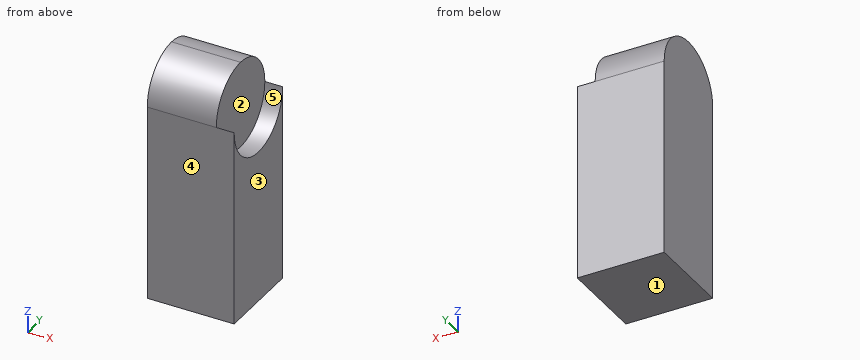
from build123d import *

# Parameters (mm, degrees)
SKETCH2_W           = 17
SKETCH2_H           = 17
BOSS_EXTRUDE1_DEPTH = 47
CUT_EXTRUDE1_DEPTH  = 47
SKETCH6_R           = 8.5
CUT_EXTRUDE3_DEPTH  = 3.5


with BuildPart() as part:
    # Sketch2 → Boss-Extrude1 (new body)
    with BuildSketch(Plane.XY):
        Rectangle(SKETCH2_W, SKETCH2_H)
    extrude(amount=BOSS_EXTRUDE1_DEPTH)

    # Sketch3 → Cut-Extrude1 (cut)
    with BuildSketch(Plane(origin=(8.5, 0, 0), x_dir=(0, 0, -1), z_dir=(1, 0, 0))):
        with BuildLine():
            Line((-38.5, 8.5), (-47, 8.5))
            Line((-47, 8.5), (-47, 0))
            ThreePointArc((-47, 0), (-44.51040764, 6.01040764), (-38.5, 8.5))
        make_face()
        with BuildLine():
            ThreePointArc((-38.5, -8.5), (-44.51040764, -6.01040764), (-47, 0))
            Line((-47, 0), (-47, -8.5))
            Line((-47, -8.5), (-38.5, -8.5))
        make_face()
    extrude(amount=-CUT_EXTRUDE1_DEPTH, mode=Mode.SUBTRACT)

    # Sketch6 → Cut-Extrude3 (cut)
    with BuildSketch(Plane(origin=(8.5, 0, 0), x_dir=(0, 0, -1), z_dir=(1, 0, 0))):
        with Locations((-38.5, 0)):
            Circle(SKETCH6_R)
    extrude(amount=-CUT_EXTRUDE3_DEPTH, mode=Mode.SUBTRACT)


solid = part.part
Read the model definition and answer for the solid it produces. Units are mm, in the model's axes. Face numbers are marked on the shaded views. A direction names the side the tool comes from. Round coordinates to 2 decimals unless told otherwise and drop trailing zeros. Write each loop counter-clockwise with the first axis right and the second up, starting at its lowest first coordinate (ties: lowest second). Pieces come first, ordered by that corner, then holes.
1. Determine the mould class of the marked faces 3, 4 and 5 for opening direction Y: pulls with the +Y half, pulls with the -Y half, needs draft (parallel to the pull), parting line crosses it, or undercut.
2. Which of the six approach directions +Z, -Z, +X, -X, +Y, -Y give full straight-line access (tool end or side, diameter ignored) to the marked faces 1 and 2?
3. Straight lines are drawn through the part: L1, parallel to X at y = 0.5, z = 40; L2, parallel to Z at x = 1, y = -2.75; L3, parallel to Z at x = 1.5, y = 3.25. For each, find the intervals that lie inside material, in ascending order.
4. Given pin 1 Ø4 at (y, z) = (-3, 39) entering from +X, flat-ended and moving along its own axis, determine where the tip first touches the part or whether it passes through.
5. The part is cut by section D-D, the plane z = 31.5. Determine the outline of the cut face in (x, y).
6. The part is cut by section B-B, the plane y = -0.5. Determine the outline of the cut face in (x, z).
7. The part is cut by section C-C, the plane x = -0.25. Determine the outline of the cut face in (y, z), then the cut area to 3 significant figures.
Values:
1. face 3: needs draft
1. face 4: pulls with the -Y half
1. face 5: undercut
2. face 1: -Z, +X, -X, +Y, -Y
2. face 2: +Z, +X
3. L1: x = -8.5 to 5
3. L2: z = 0 to 46.54
3. L3: z = 0 to 46.35
4. pin 1: stops at x = 5
5. outline: (-8.5, -8.5) - (8.5, -8.5) - (8.5, -4.82) - (5, -4.82) - (5, 4.82) - (8.5, 4.82) - (8.5, 8.5) - (-8.5, 8.5) - close
6. outline: (-8.5, 0) - (8.5, 0) - (8.5, 30.01) - (5, 30.01) - (5, 46.99) - (-8.5, 46.99) - close
7. outline: (-8.5, 0) - (8.5, 0) - (8.5, 38.5) arc R8.5 ccw to (-8.5, 38.5) - close
7. area: 768 mm2
